```python
from build123d import *

# Parameters (mm, degrees)
SKETCH2_R           = 12
BOSS_EXTRUDE1_DEPTH = 4
SKETCH3_R           = 8
BOSS_EXTRUDE2_DEPTH = 105
FILLET1_R           = 1
FILLET2_R           = 1
SKETCH4_R           = 2
CUT_EXTRUDE1_DEPTH  = 10


with BuildPart() as part:
    # Sketch2 → Boss-Extrude1 (new body, symmetric)
    with BuildSketch(Plane(origin=(0, 0, 0), x_dir=(0, 0, -1), z_dir=(1, 0, 0))):
        Circle(SKETCH2_R)
    extrude(amount=BOSS_EXTRUDE1_DEPTH, both=True)

    # Sketch3 → Boss-Extrude2 (add)
    with BuildSketch(Plane(origin=(4, 0, 0), x_dir=(0, 0, -1), z_dir=(1, 0, 0))):
        Circle(SKETCH3_R)
    extrude(amount=BOSS_EXTRUDE2_DEPTH)

    # Fillet1
    fillet1_edges = [part.edges().sort_by_distance(p)[0] for p in [
        (-4, 0, 12),
    ]]
    fillet(fillet1_edges, radius=FILLET1_R)

    # Fillet2
    fillet2_edges = [part.edges().sort_by_distance(p)[0] for p in [
        (109, 0, 8),
    ]]
    fillet(fillet2_edges, radius=FILLET2_R)

    # Sketch4 → Cut-Extrude1 (cut, symmetric)
    with BuildSketch(Plane.XY):
        with Locations((98, 0)):
            Circle(SKETCH4_R)
    extrude(amount=CUT_EXTRUDE1_DEPTH, both=True, mode=Mode.SUBTRACT)


solid = part.part
```
Check sheet for the modelled part. Datum: model origin and axes. Units: mm. A direction names the side the tool comes from. Round coordinates to 2 decimals unless told otherwise and drop trailing zeros. Order: outer loops, then holes, each group sorted by start corner. A loop starts at its lowest first (then second) coordinate and runs counter-clockwise, first axis right, second up. Notation, with made-up numbers: (74.5, 64.25) -> (79.5, 64.25) arc R16 ccw to (79.5, 91.25) -> close; hole circle Ø1 at (25.25, 87.25). An arc over 180 degrees is marked (long way). One line per item, written item: value. Start each with the question number.
Q1. Thickness scan on line 1 (X direction, y = 0, z = 2); line 2 (X direction, y = 3, z = -8.75); line 3 (Y direction, x = 104, z = -0.5). Record the ranges inside material, lowest first.
Q2. Cross-section at C-C (x = 98). Record the boundary of the cut face in (y, z).
Q3. Gauge pin test, flat ends, axial feed: pin 1 Ø5 at (x, y) = (74, 5) entering from -Z; pin 2 Ø3 at (x, z) = (21, 4.5) entering from -Y; pin 3 Ø5 at (x, z) = (47.5, 0.5) entering from -Y. Record the tip position at first contact, or that the pin passes through.
Q4. Cross-section at D-D (x = 13). Record the boundary of the cut face in (y, z).
Q5. Mould release check, pull along X, two halves, no side actions. Record for faces 3 (the face through (4, -8, -2)), 4 (the face through (99.908, 0.601, 0.112)), 5 (the face through (0.55, 0.53, 11.99)): pulls with the +X half, pulls with the -X half, needs draft (parallel to the pull), parting line crosses it, or undercut.
Q6. Cross-section at A-A (y = 0). Record the boundary of the cut face in (x, z).
Q7. Cross-section at B-B (z = 0). Record the boundary of the cut face in (x, y).
Q8. Set-up check for faces 1 (the face through (109, 0, 0)), 2 (the face through (55.27, -7.81, 1.73)): record each of +Z, -Z, +X, -X, +Y, -Y from which the full face is reachable in a straight line by a thin tool's end or side.
Completed:
1. line 1: x = -4 to 96, 100 to 109
1. line 2: x = -4 to 4
1. line 3: y = -7.98 to 7.98
2. outline: (-2, -7.75) -> (-2, 7.75) arc R8 ccw to start; (2, -7.75) arc R8 ccw to (2, 7.75) -> close
3. pin 1: stops at z = -7.6
3. pin 2: stops at y = -7.42
3. pin 3: stops at y = -8
4. outline: circle Ø16 at (0, 0)
5. face 3: pulls with the +X half
5. face 4: undercut
5. face 5: needs draft
6. outline: (-4, -11) arc R1 ccw to (-3, -12) -> (4, -12) -> (4, -8) -> (96, -8) -> (96, 8) -> (4, 8) -> (4, 12) -> (-3, 12) arc R1 ccw to (-4, 11) -> close; (100, -8) -> (108, -8) arc R1 ccw to (109, -7) -> (109, 7) arc R1 ccw to (108, 8) -> (100, 8) -> close
7. outline: (-4, -11) arc R1 ccw to (-3, -12) -> (4, -12) -> (4, -8) -> (108, -8) arc R1 ccw to (109, -7) -> (109, 7) arc R1 ccw to (108, 8) -> (4, 8) -> (4, 12) -> (-3, 12) arc R1 ccw to (-4, 11) -> close; hole circle Ø4 at (98, 0)
8. face 1: +Z, -Z, +X, +Y, -Y
8. face 2: +X
